Build history of the part. All positions in model axes, mm. Face numbers are marked on the shaded views. A direction names the side the tool comes from. Give positions to 0.01 mm unless a question says otherwise; leave off trailing zeros. Loops run counter-clockwise (first coordinate to the right, second up) from the corner with the lowest first, then second, coordinate; pieces in that order, holes last. Notation, with made-up numbers: M 69,38 L 112,38 A16 ccw 112,48 Z; hole C 29,64 d5. An arc over 180 degrees is marked long. Answer in a Markdown table with one row per item. Add a question column.
```python
from build123d import *

# Parameters (mm, degrees)
F1_DEPTH = 6.35
F2_SIZE  = 5.08
F3_R     = 1.27
F4_R     = 0.508


with BuildPart() as f1:
    # F0 (on Top) → F1 (new body)
    with BuildSketch(Plane.XY):
        with BuildLine():
            Line((0, 25.4), (0, 0))
            Line((0, 0), (9.525, 0))
            Line((9.525, 0), (9.525, 25.4))
            ThreePointArc((9.525, 25.4), (14.4145, 30.2895), (19.304, 25.4))
            Line((19.304, 25.4), (19.304, 12.7))
            Line((19.304, 12.7), (28.829, 12.7))
            Line((28.829, 12.7), (28.829, 25.4))
            ThreePointArc((28.829, 25.4), (14.4145, 39.8145), (0, 25.4))
        make_face()
    extrude(amount=F1_DEPTH)

    # F2
    f2_edges = [f1.edges().sort_by_distance(p)[0] for p in [
        (28.829, 12.7, 3.175),
    ]]
    chamfer(f2_edges, length=F2_SIZE)

    # F3
    f3_edges = [f1.edges().sort_by_distance(p)[0] for p in [
        (23.749, 12.7, 3.175),
        (28.829, 17.78, 3.175),
        (19.304, 12.7, 3.175),
        (0, 0, 3.175),
        (9.525, 0, 3.175),
    ]]
    fillet(f3_edges, radius=F3_R)

    # F4
    f4_edges = [f1.edges().sort_by_distance(p)[0] for p in [
        (21.898474, 12.7, 6.35),
        (19.675974, 13.071974, 6.35),
        (23.708957, 12.796673, 6.35),
        (19.304, 19.685, 6.35),
        (26.289, 15.24, 6.35),
        (14.4145, 30.2895, 6.35),
        (28.732327, 17.820043, 6.35),
        (9.525, 13.335, 6.35),
        (28.829, 21.853026, 6.35),
        (9.153026, 0.371974, 6.35),
        (14.4145, 39.8145, 6.35),
        (4.7625, 0, 6.35),
        (0, 13.335, 6.35),
        (0.371974, 0.371974, 6.35),
        (21.898474, 12.7, 0),
        (19.675974, 13.071974, 0),
        (23.708957, 12.796673, 0),
        (19.304, 19.685, 0),
        (26.289, 15.24, 0),
        (14.4145, 30.2895, 0),
        (28.732327, 17.820043, 0),
        (9.525, 13.335, 0),
        (28.829, 21.853026, 0),
        (9.153026, 0.371974, 0),
        (14.4145, 39.8145, 0),
        (4.7625, 0, 0),
        (0, 13.335, 0),
        (0.371974, 0.371974, 0),
    ]]
    fillet(f4_edges, radius=F4_R)


solid = f1.part
```
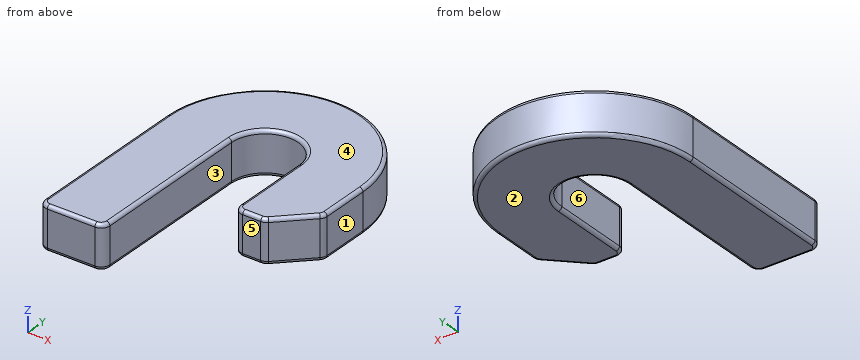
(1) Pin check, flat tips, straight feed: pin 1 (1.3 mm diameter, centred on x = 21.5, z = 2, fed in from -Y); pin 2 (1.6 mm diameter, centred on y = 11, z = 4.5, fed in from +X) (3 decimals). Stop position of each tip, or through.
(2) Slice it at A-A, the plane y = 22. Give the cut face in (x, z) (3 decimals), then the cut area to 3 significant figures.
(3) Slice it at C-C, the plane y = 4. Give the cut face in (x, z) (3 decimals), then the cut area to 3 significant figures.
(4) Slice it at B-B, the plane z = 4.5. Give the cut face in (x, y) (1 decimal).
(5) Pull direction X, two halves, no side cores. Call the marked faces 1, 2 and 3: +X half, -X half, draft (parallel to the pull), parting line (faces both ways), or undercut.
(6) Tool access for the marked faces 4, 5 and 6: list every direction of +Z, -Z, +X, -X, +Y, -Y with a clear straight run to the whole face (end or side of a thin tool).
(7) Wall check: line 1 (X direction, y = 9, z = 4) (3 decimals); line 2 (X direction, y = 15, z = 6); line 3 (X direction, y = 14.5, z = 1) (3 decimals). Give the ranges that are in metal, low to high.
Solution:
| question | item | result |
|---|---|---|
| 1 | pin 1 | y = 12.7 |
| 1 | pin 2 | x = 9.525 |
| 2 | outline | M 0,0.508 A0.508 ccw 0.508,0 L 9.017,0 A0.508 ccw 9.525,0.508 L 9.525,5.842 A0.508 ccw 9.017,6.35 L 0.508,6.35 A0.508 ccw 0,5.842 Z; M 19.304,0.508 A0.508 ccw 19.812,0 L 28.321,0 A0.508 ccw 28.829,0.508 L 28.829,5.842 A0.508 ccw 28.321,6.35 L 19.812,6.35 A0.508 ccw 19.304,5.842 Z |
| 2 | area | 121 mm^2 |
| 3 | outline | M 0,0.508 A0.508 ccw 0.508,0 L 9.017,0 A0.508 ccw 9.525,0.508 L 9.525,5.842 A0.508 ccw 9.017,6.35 L 0.508,6.35 A0.508 ccw 0,5.842 Z |
| 3 | area | 60.3 mm^2 |
| 4 | outline | M 0,1.3 A1.3 ccw 1.3,0 L 8.3,0 A1.3 ccw 9.5,1.3 L 9.5,25.4 A4.9 cw 19.3,25.4 L 19.3,14 A1.3 ccw 20.6,12.7 L 23.2,12.7 A1.3 ccw 24.1,13.1 L 28.5,17.4 A1.3 ccw 28.8,18.3 L 28.8,25.4 A14.4 ccw 0,25.4 Z |
| 5 | face 1 | +X half |
| 5 | face 2 | draft |
| 5 | face 3 | undercut |
| 6 | face 4 | +Z, +X, -X, +Y, -Y |
| 6 | face 5 | +Z, -Z, +X, -Y |
| 6 | face 6 | +Z, -Z, -Y |
| 7 | line 1 | 0 to 9.525 |
| 7 | line 2 | 0.03 to 9.5, 19.33 to 26.01 |
| 7 | line 3 | 0 to 9.525, 19.304 to 25.549 |
